Answer from the drawing. Dimensions are ordinates in mm from the lowest x, y and z of the part. A direction names the side the tool comes from. Give positions to 0.01 mm unless a question says otherwise; leave off trailing zeros. Order: outer loops, then holes, each group sorted by start corner. A loop starts at its lowest first (then second) coordinate and runs counter-clockwise, first axis right, second up. Notation, with made-up numbers: (81.5, 22) - (93.5, 22) arc R22 ccw to (93.5, 53) - close; hole circle Ø4 at (55, 34). An arc over 180 degrees is marked (long way). Write each question's results on one line, items separated by ' | '.
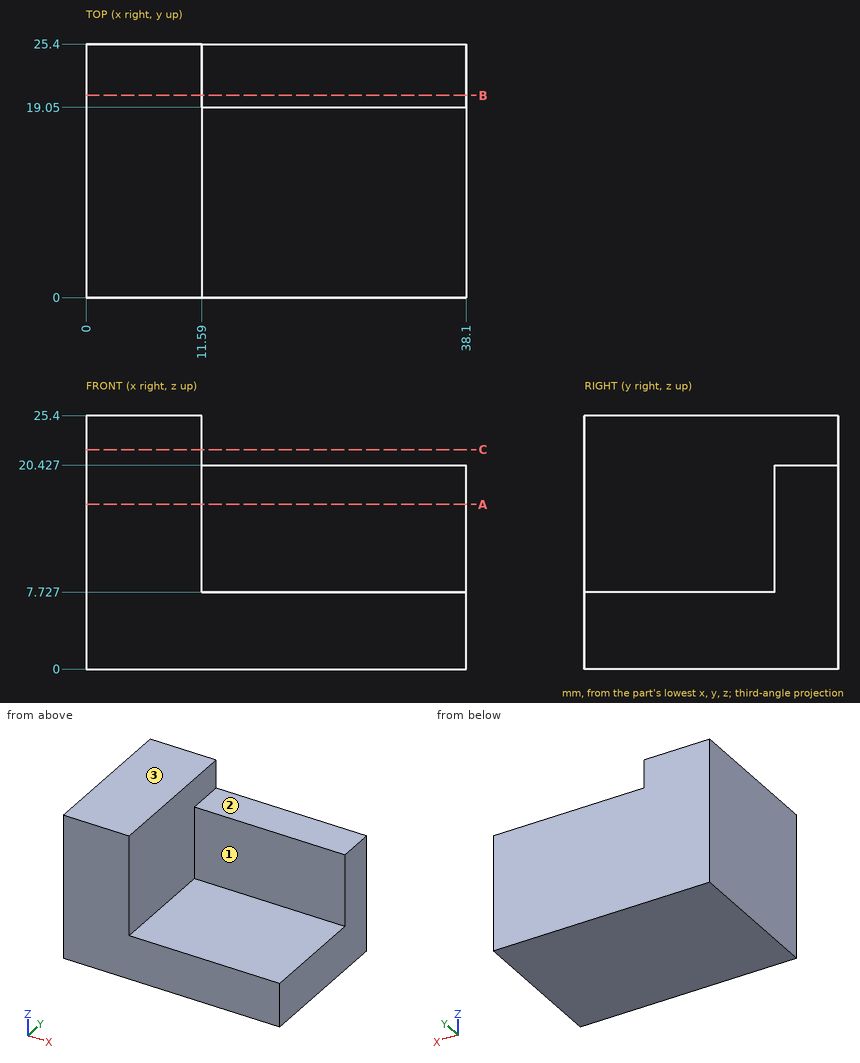
(1) Consider probe 1 along X at (y, z) = (13, 10.25); probe 2 along Y at (x, z) = (31, 12.5); probe 3 along Z at (x, y) = (29.5, 16.75). Determine where each line is inside the solid, lowest interval first. Write a range as [from, to].
Conclusion:
probe 1: [0, 11.59] | probe 2: [19.05, 25.4] | probe 3: [0, 7.73]
(2) Each of these flat-tipped pins is pushed along its axis until it touches: pin 1 (10 mm diameter, centred on y = 8, z = 17, fed in from +X); pin 2 (1.9 mm diameter, centred on x = 26.5, y = 22.5, fed in from +Z); pin 3 (12 mm diameter, centred on x = 24.5, z = 19.5, fed in from -Y). Where does it stop, or does it pass through?
Conclusion:
pin 1: x = 11.59 | pin 2: z = 20.43 | pin 3: y = 19.05
(3) For the marked faces 1, 2 and 3, determine the directions among +Z, -Z, +X, -X, +Y, -Y from which every point of the face is accessible in a straight line to the end or side of a thin tool.
Conclusion:
face 1: +Z, +X, -Y | face 2: +Z, +X, +Y, -Y | face 3: +Z, +X, -X, +Y, -Y
(4) Section B-B (y = 20.25) is taken. Give the vertices of the cut face in (x, z).
Conclusion:
outline: (0, 0) - (38.1, 0) - (38.1, 20.43) - (11.59, 20.43) - (11.59, 25.4) - (0, 25.4) - close
(5) Section A-A (z = 16.5) is taken. Give the vertices of the cut face in (x, y).
Conclusion:
outline: (0, 0) - (11.59, 0) - (11.59, 19.05) - (38.1, 19.05) - (38.1, 25.4) - (0, 25.4) - close
(6) Section C-C (z = 22) is taken. Give the vertices of the cut face in (x, y), plus the area to 3 significant figures.
Conclusion:
outline: (0, 0) - (11.59, 0) - (11.59, 25.4) - (0, 25.4) - close | area: 294 mm^2
